Check sheet for the modelled part. Datum: model origin and axes. Units: mm. Face numbers are marked on the shaded views. Give positions to 0.01 mm unless a question says otherwise; leave off trailing zeros. Loops run counter-clockwise (first coordinate to the right, second up) from the corner with the lowest first, then second, coordinate; pieces in that order, holes last. Notation, with made-up numbers: (61, -37.5) - (97, -37.5) arc R29 ccw to (97, -10.5) - close; hole circle Ø4 at (-10.75, 7). An arc over 180 degrees is marked (long way). Use CSV: the item, a comma, the result in double quotes.
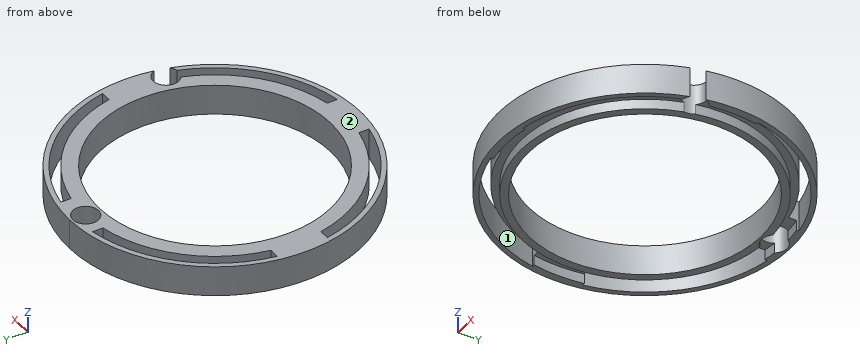
from build123d import *

# Parameters (mm, degrees)
CUT_EXTRUDE1_DEPTH = 7
SKETCH4_R          = 2.55
CUT_EXTRUDE2_DEPTH = 7


with BuildPart() as part:
    # Sketch2 → Revolve1 (revolve)
    with BuildSketch(Plane.ZY.offset(-259.301545348)):
        Polygon((0, -124.073704322), (0, -125.573704322), (6, -125.573704322), (6, -119.573704322), (0, -119.573704322), (0, -121.073704322), (2, -121.073704322), (2, -124.073704322), align=None)
    revolve(axis=Axis((259.301545348, -148.573704322, 22.865), (0, 0, 1)))

    # Sketch3 → Cut-Extrude1 (cut, through all)
    with BuildSketch(Plane.XY.offset(6)):
        with BuildLine():
            Line((254.301545348, -174.088405967), (254.301545348, -176.12365895))
            ThreePointArc((254.301545348, -176.12365895), (239.502555475, -168.372694195), (231.75159072, -153.573704322))
            Line((231.75159072, -153.573704322), (233.786843704, -153.573704322))
            ThreePointArc((233.786843704, -153.573704322), (240.916769037, -166.958480633), (254.301545348, -174.088405967))
        make_face()
        with BuildLine():
            Line((264.301545348, -174.088405967), (264.301545348, -176.12365895))
            ThreePointArc((264.301545348, -176.12365895), (279.100535221, -168.372694195), (286.851499976, -153.573704322))
            Line((286.851499976, -153.573704322), (284.816246992, -153.573704322))
            ThreePointArc((284.816246992, -153.573704322), (277.686321659, -166.958480633), (264.301545348, -174.088405967))
        make_face()
        with BuildLine():
            Line((286.851499976, -143.573704322), (284.816246992, -143.573704322))
            ThreePointArc((284.816246992, -143.573704322), (277.686321659, -130.188928011), (264.301545348, -123.059002678))
            Line((264.301545348, -123.059002678), (264.301545348, -121.023749694))
            ThreePointArc((264.301545348, -121.023749694), (279.100535221, -128.774714449), (286.851499976, -143.573704322))
        make_face()
        with BuildLine():
            Line((254.301545348, -121.023749694), (254.301545348, -123.059002678))
            ThreePointArc((254.301545348, -123.059002678), (240.916769037, -130.188928011), (233.786843704, -143.573704322))
            Line((233.786843704, -143.573704322), (231.75159072, -143.573704322))
            ThreePointArc((231.75159072, -143.573704322), (239.502555475, -128.774714449), (254.301545348, -121.023749694))
        make_face()
    extrude(amount=-CUT_EXTRUDE1_DEPTH, mode=Mode.SUBTRACT)

    # Sketch4 → Cut-Extrude2 (cut, through all)
    with BuildSketch(Plane.XY.offset(6)):
        with Locations((258.944661735, -122.573704322)):
            Circle(SKETCH4_R)
        with Locations((285.301545348, -155.216820709)):
            Circle(SKETCH4_R)
        with Locations((252.658428961, -181.573704322)):
            Circle(SKETCH4_R)
        with Locations((226.301545348, -148.930587935)):
            Circle(SKETCH4_R)
    extrude(amount=-CUT_EXTRUDE2_DEPTH, mode=Mode.SUBTRACT)


solid = part.part
1. Sectioned sample at D-D, the plane y = -149.5. Record the boundary of the cut face in (x, z), and give its area (3 significant figures).
Completed:
outline,"(230.32, 0) - (231.82, 0) - (231.82, 2) - (234.82, 2) - (234.82, 0) - (236.32, 0) - (236.32, 6) - (230.32, 6) - close; (282.28, 0) - (283.78, 0) - (283.78, 2) - (286.79, 2) - (286.79, 0) - (288.29, 0) - (288.29, 6) - (282.28, 6) - close"
area,"60.0 mm²"
2. Sectioned sample at A-A, the plane y = -135. Record the boundary of the cut face in (x, z).
Completed:
outline,"(233.67, 0) - (234.81, 0) - (234.81, 6) - (233.67, 6) - close; (237.13, 2) - (238.91, 2) - (238.91, 0) - (240.73, 0) - (240.73, 6) - (237.13, 6) - close; (277.87, 0) - (279.7, 0) - (279.7, 2) - (281.48, 2) - (281.48, 6) - (277.87, 6) - close; (283.79, 0) - (284.93, 0) - (284.93, 6) - (283.79, 6) - close"
3. Sectioned sample at B-B, the plane x = 278. Record the boundary of the cut face in (y, z), and give its area (3 significant figures).
Completed:
outline,"(-170.74, 0) - (-169.42, 0) - (-169.42, 6) - (-170.74, 6) - close; (-166.64, 2) - (-164.4, 2) - (-164.4, 0) - (-161.97, 0) - (-161.97, 6) - (-166.64, 6) - close; (-135.18, 0) - (-132.74, 0) - (-132.74, 2) - (-130.51, 2) - (-130.51, 6) - (-135.18, 6) - close; (-127.73, 0) - (-126.41, 0) - (-126.41, 6) - (-127.73, 6) - close"
area,"63.0 mm²"
4. Release check for a two-part mould opening along X. For the marked faces 1 and 2 record: released by +X, released by -X, zero draft, split by the parting line, or undercut.
Completed:
face 1,"undercut"
face 2,"zero draft"
5. Sectioned sample at C-C, the plane z = 3. Record the boundary of the cut face in (x, y).
Completed:
outline,"(264.3, -176.12) - (264.3, -174.09) arc R26 ccw to (283.8, -157.28) arc R2.55 cw (long way) to (287.71, -154.39) arc R29 ccw (long way) to (287.02, -157.1) arc R2.55 cw to (285.76, -157.72) arc R28 cw to start; hole (231.75, -153.57) arc R28 ccw to (254.3, -176.12) - (254.3, -174.09) arc R26 cw to (233.79, -153.57) - close; hole (231.75, -143.57) - (233.79, -143.57) arc R26 cw to (254.3, -123.06) - (254.3, -121.02) arc R28 ccw to start; hole circle Ø46 at (259.3, -148.57); hole circle Ø5.1 at (258.94, -122.57); hole (264.3, -123.06) arc R26 cw to (284.82, -143.57) - (286.85, -143.57) arc R28 ccw to (264.3, -121.02) - close"
6. Go/stop test with flat-tipped pins: pin 1 Ø1.6 at (x, z) = (286, 3.5) entering from +Y; pin 2 Ø1.6 at (y, z) = (-121.5, 3.5) entering from +X; pin 3 Ø0.6 at (y, z) = (-122.5, 4) entering from -X; pin 4 Ø3 at (x, y) = (285.3, -155.22) entering from -Z. Record where each tip stops, or that it passes through.
Completed:
pin 1,"stops at y = -135.52"
pin 2,"stops at x = 271.58"
pin 3,"stops at x = 246.01"
pin 4,"passes through"
7. Scan lines: line 1 along X through (y, z) = (-148, 1.4); line 2 along Y through (x, z) = (259, 4.4); line 3 along Y through (x, z) = (242, 0.95). Record each from-to range of solid material in increasing order.
Completed:
line 1,"x = 230.31 to 231.81, 234.81 to 236.31, 282.29 to 283.79, 286.8 to 288.3"
line 2,"y = -177.57 to -171.57, -125.58 to -125.12, -120.02 to -119.58"
line 3,"y = -171.85 to -170.59, -165.92 to -163.73, -133.42 to -131.23, -126.56 to -125.3"
